Could you check a few things on this model? Use its own coordinates, in mm. Face numbers are marked on the shaded views. A direction names the side the tool comes from. Coordinates: 2 decimals unless noted, no trailing zeros. Loops run counter-clockwise (first coordinate to the right, second up) from the corner with the lowest first, then second, coordinate; pieces in that order, holes last. Notation, with made-up numbers: M 3.5,-22.5 L 52.5,-22.5 A7 ccw 52.5,-12.5 Z; hole C 78,63.25 d2. An arc over 180 degrees is marked long. Use one line per item in the form item = value. Start each with the question number.
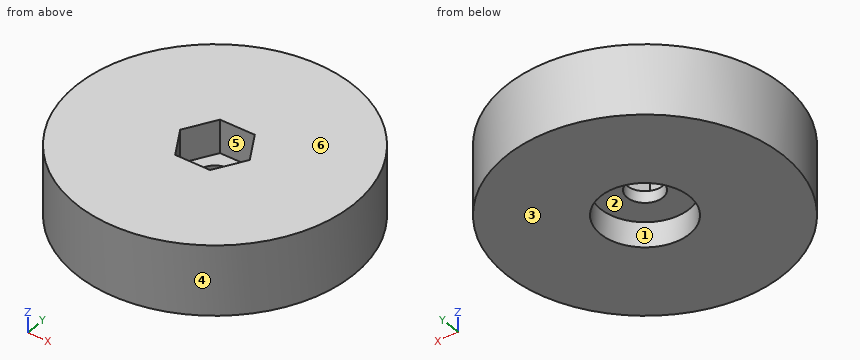
```python
from build123d import *

# Parameters (mm, degrees)
BOX027_W          = 40
BOX027_H          = 50
BOX027_DEPTH      = 0.7
CYLINDER062_R     = 4
CYLINDER062_DEPTH = 2.75
CYLINDER019_R     = 1.6
CYLINDER019_DEPTH = 22.75
CYLINDER018_R     = 4
CYLINDER018_DEPTH = 2.75
PRISM003_DEPTH    = 3
CYLINDER017_R     = 12.5
CYLINDER017_DEPTH = 7


with BuildPart() as cube027:
    # Box027 → Box027 (new body)
    with BuildSketch(Plane(origin=(-10, 0, 15), x_dir=(1, 0, 0), z_dir=(0, 0, 1))):
        with Locations((20, 25)):
            Rectangle(BOX027_W, BOX027_H)
    extrude(amount=BOX027_DEPTH)


with BuildPart() as cylinder062:
    # Cylinder062 → Cylinder062 (new body)
    with BuildSketch(Plane(origin=(10, 20, 15.2), x_dir=(1, 0, 0), z_dir=(0, 0, 1))):
        Circle(CYLINDER062_R)
    extrude(amount=CYLINDER062_DEPTH)


with BuildPart() as cylinder018:
    # Cylinder019 → Cylinder019 (new body)
    with BuildSketch(Plane(origin=(10, 0, -31), x_dir=(1, 0, 0), z_dir=(0, 0, 1))):
        Circle(CYLINDER019_R)
    extrude(amount=CYLINDER019_DEPTH)


with BuildPart() as cylinder017:
    # Cylinder018 → Cylinder018 (new body)
    with BuildSketch(Plane(origin=(10, 0, -27), x_dir=(1, 0, 0), z_dir=(0, 0, 1))):
        Circle(CYLINDER018_R)
    extrude(amount=CYLINDER018_DEPTH)


with BuildPart() as prism003:
    # Prism003 → Prism003 (new body)
    with BuildSketch(Plane(origin=(10, 0, -20), x_dir=(1, 0, 0), z_dir=(0, 0, -1))):
        Polygon((3.15, 0), (1.575, 2.72798), (-1.575, 2.72798), (-3.15, 0), (-1.575, -2.72798), (1.575, -2.72798), align=None)
    extrude(amount=PRISM003_DEPTH)


with BuildPart() as plato_tornillo001:
    # Cylinder017 → Cylinder017 (new body)
    with BuildSketch(Plane(origin=(10, 0, -27), x_dir=(1, 0, 0), z_dir=(0, 0, 1))):
        Circle(CYLINDER017_R)
    extrude(amount=CYLINDER017_DEPTH)

    # Cut014: cut Prism003
    add(prism003.part, mode=Mode.SUBTRACT)

    # Cut015: cut Cylinder017
    add(cylinder017.part, mode=Mode.SUBTRACT)

    # Cut016: cut Cylinder018
    add(cylinder018.part, mode=Mode.SUBTRACT)


with BuildPart() as plato_tornillo001_1:
    # Cut016 placement: moved
    add(plato_tornillo001.part.moved(Location((0, 20, 42))))

    # Cut049: cut Cylinder062
    add(cylinder062.part, mode=Mode.SUBTRACT)

    # Cut050: cut Cube027
    add(cube027.part, mode=Mode.SUBTRACT)


solid = plato_tornillo001_1.part
```
Item 1: For the marked faces 5 and 6, which set-ups out of +Z, -Z, +X, -X, +Y, -Y let a thin tool reach every point of the face, with its end or its side?
Item 2: I want a section at B-B (z = 20.25). Write out the boundary of the cut face in (x, y) (3 decimals).
Item 3: Please list where these lines run through material, in increasing order: line 1 along Y through (x, z) = (10, 16.7); line 2 along X through (y, z) = (20, 18.5); line 3 along Y through (x, z) = (10, 18.5).
Item 4: Thinking about a two-plate mould opening in X: for the marked faces 1, 2, 3 and 4, which applies, pulls with the +X half, pulls with the -X half, needs draft (parallel to the pull), parting line crosses it, or undercut?
Item 5: I want a section at C-C (x = 0). Write out the boundary of the cut face in (y, z).
Item 6: I want a section at D-D (y = 29.5). Write out the boundary of the cut face in (x, z).
Item 7: I'm going to push flat-ended pins straight in: P1, Ø2.5, axis at x = 10, y = 20, coming from the -Z side; P2, Ø1.5, axis at x = 9.5, z = 21, coming from the +Y side; P3, Ø2.5, axis at x = 9, y = 19, coming from the -Z side; P4, Ø2.5, axis at x = 9.5, y = 21, coming from the +Z side. Where does each tip first touch, or does it pass through?
Item 8: I want a section at A-A (x = 10). Write out the boundary of the cut face in (y, z).
Worked answers:
q1.face_5 = +Z
q1.face_6 = +Z, +X, -X, +Y, -Y
q2.outline = C 10,20 d25; hole M 6.85,20 L 8.425,17.272 L 11.575,17.272 L 13.15,20 L 11.575,22.728 L 8.425,22.728 Z
q3.line_1 = 7.5 to 16, 24 to 32.5
q3.line_2 = -2.5 to 8.4, 11.6 to 22.5
q3.line_3 = 7.5 to 18.4, 21.6 to 32.5
q4.face_1 = undercut
q4.face_2 = undercut
q4.face_3 = needs draft
q4.face_4 = parting line crosses it
q5.outline = M 12.5,15.7 L 27.5,15.7 L 27.5,22 L 12.5,22 Z
q6.outline = M 1.88,15.7 L 18.12,15.7 L 18.12,22 L 1.88,22 Z
q7.P1 = through
q7.P2 = 32.5
q7.P3 = 17.95
q7.P4 = 19
q8.outline = M 7.5,15.7 L 16,15.7 L 16,17.95 L 18.4,17.95 L 18.4,19 L 17.27,19 L 17.27,22 L 7.5,22 Z; M 21.6,17.95 L 24,17.95 L 24,15.7 L 32.5,15.7 L 32.5,22 L 22.73,22 L 22.73,19 L 21.6,19 Z
